from build123d import *

# Parameters (mm, degrees)
SKETCH1_R           = 74.18267629
BOSS_EXTRUDE2_DEPTH = 3
SKETCH1_4_R         = 17.5
SKETCH1_4_R_2       = 10
CUT_EXTRUDE1_DEPTH  = 4
SKETCH1_5_R         = 2.5
CUT_EXTRUDE2_DEPTH  = 4


with BuildPart() as part:
    # Sketch1 → Boss-Extrude2 (new body)
    with BuildSketch(Plane(origin=(0, 0, 0), x_dir=(1, 0, 0), z_dir=(0, 1, 0))):
        Circle(SKETCH1_R)
    extrude(amount=-BOSS_EXTRUDE2_DEPTH)

    # Sketch1<4> → Cut-Extrude1 (cut)
    with BuildSketch(Plane(origin=(0, 0, 0), x_dir=(1, 0, 0), z_dir=(0, 1, 0))):
        with Locations((0, 48.18267629)):
            Circle(SKETCH1_4_R)
        with Locations((45.824448258, 14.889265808)):
            Circle(SKETCH1_4_R)
        with Locations((28.321066539, -38.980603953)):
            Circle(SKETCH1_4_R)
        with Locations((-28.321066539, -38.980603953)):
            Circle(SKETCH1_4_R)
        with Locations((-45.824448258, 14.889265808)):
            Circle(SKETCH1_4_R)
        Circle(SKETCH1_4_R_2)
    extrude(amount=-CUT_EXTRUDE1_DEPTH, mode=Mode.SUBTRACT)

    # Sketch1<5> → Cut-Extrude2 (cut)
    with BuildSketch(Plane(origin=(0, 0, 0), x_dir=(1, 0, 0), z_dir=(0, 1, 0))):
        with Locations((40.958449464, 56.374469332)):
            Circle(SKETCH1_5_R)
        with Locations((66.272163358, -21.533131187)):
            Circle(SKETCH1_5_R)
        with Locations((0, -69.68267629)):
            Circle(SKETCH1_5_R)
        with Locations((-66.605033139, -21.641287135)):
            Circle(SKETCH1_5_R)
        with Locations((-40.958449464, 56.374469332)):
            Circle(SKETCH1_5_R)
    extrude(amount=-CUT_EXTRUDE2_DEPTH, mode=Mode.SUBTRACT)


solid = part.part
Verification items for the finished model (mm, model axes). Give positions to 0.01 mm unless a question says otherwise; leave off trailing zeros. Loops run counter-clockwise (first coordinate to the right, second up) from the corner with the lowest first, then second, coordinate; pieces in that order, holes last.
1) Depth check by flat-ended pin: pin 1 Ø3 at (x, z) = (40.96, -56.37) entering from -Y; pin 2 Ø1.5 at (y, z) = (-0.5, -45.5) entering from +X. Enter the tip coordinate at first touch or a pass-through.
2) Sectioned sample at B-B, the plane z = -38. Enter the section's corners in (x, y), then the cut area to 3 significant figures.
3) Sectioned sample at C-C, the plane x = 47.5. Enter the section's corners in (y, z), then the cut area to 3 significant figures.
4) Draft check along X on faces 1 (the cylindrical face through (34.231, -1.479, 65.813)), 2 (the flat face through (15, -3, -1)), 3 (the cylindrical face through (26.04, -1.48, 21.63)). Enter one of: pulls with the +X half, pulls with the -X half, needs draft (parallel to the pull), parting line crosses it, or undercut.
5) Sectioned sample at D-D, the plane z = -22. Enter the section's corners in (x, y), then the cut area to 3 significant figures.
6) Thickness scan on line 1 along Z through (x, y) = (0, -1.2); line 2 along Z through (x, y) = (13, -1); line 3 along Z through (x, y) = (-15.5, -0.95). Record the ranges inside material, lowest first.
7) Sectioned sample at A-A, the plane x = 0. Enter the section's corners in (y, z).
Answers:
1. pin 1: passes through
1. pin 2: stops at x = 59.17
2. outline: (-63.71, -3) - (-14.23, -3) - (-14.23, 0) - (-63.71, 0) - close; (14.23, -3) - (63.71, -3) - (63.71, 0) - (14.23, 0) - close
2. area: 297 mm2
3. outline: (-3, -56.98) - (0, -56.98) - (0, -32.31) - (-3, -32.31) - close; (-3, 2.53) - (0, 2.53) - (0, 56.98) - (-3, 56.98) - close
3. area: 237 mm2
4. face 1: parting line crosses it
4. face 2: needs draft
4. face 3: undercut
5. outline: (-70.85, -3) - (-61.81, -3) - (-61.81, 0) - (-70.85, 0) - close; (-29.83, -3) - (29.83, -3) - (29.83, 0) - (-29.83, 0) - close; (61.81, -3) - (70.85, -3) - (70.85, 0) - (61.81, 0) - close
5. area: 233 mm2
6. line 1: z = -74.18 to -65.68, -30.68 to -10, 10 to 67.18, 72.18 to 74.18
6. line 2: z = -73.03 to -59.9, -36.47 to 30.52, 47.44 to 73.03
6. line 3: z = -72.55 to -56.31, -40.06 to 27.07, 50.89 to 72.55
7. outline: (-3, -74.18) - (0, -74.18) - (0, -65.68) - (-3, -65.68) - close; (-3, -30.68) - (0, -30.68) - (0, -10) - (-3, -10) - close; (-3, 10) - (0, 10) - (0, 67.18) - (-3, 67.18) - close; (-3, 72.18) - (0, 72.18) - (0, 74.18) - (-3, 74.18) - close
